Check sheet for the drawn part. Datum: minimum x, y, z corner. Units: mm. A direction names the side the tool comes from. Coordinates: 2 decimals unless noted, no trailing zeros. Loops run counter-clockwise (first coordinate to the right, second up) from the corner with the lowest first, then second, coordinate; pieces in that order, holes last.
Q1. Sectioned sample at C-C (x = 83). Enter the section's corners in (y, z).
Q2. Access from +Z, -Z, +X, -X, +Y, -Y to the whole of each face (thin tool, end or side, straight path). Record for the marked faces 5, 6 and 7.
Q3. Sectioned sample at D-D (x = 43.5). Enter the section's corners in (y, z).
Q4. Sectioned sample at A-A (z = 4). Enter the section's corners in (x, y), then the cut area to 3 significant figures.
Q5. Sectioned sample at B-B (y = 16.5). Enter the section's corners in (x, z), then the cut area to 3 significant figures.
Q6. Mould release check, pull along Z, two halves, no side actions. Record for the marked faces 1, 2, 3 and 4: +Z half, -Z half, draft (parallel to the pull), parting line (faces both ways), or undercut.
Q7. Material ranges on probe 1 along X at (y, z) = (1.3, 59); probe 2 along Z at (x, y) = (83, 1.75); probe 3 along Z at (x, y) = (73.5, 5.5), recorded low to high.
Q8. Go/stop test with flat-tipped pins: P1, Ø2.5, axis at x = 33.5, z = 4.5, coming from the +Y side; P2, Ø12, axis at y = 7.5, z = 49.5, coming from the -X side; P3, Ø1, axis at x = 68, y = 9, coming from the +Z side; P4, Ø8, axis at x = 38, z = 27, coming from the -Y side. Record where each tip stops, or that it passes through.
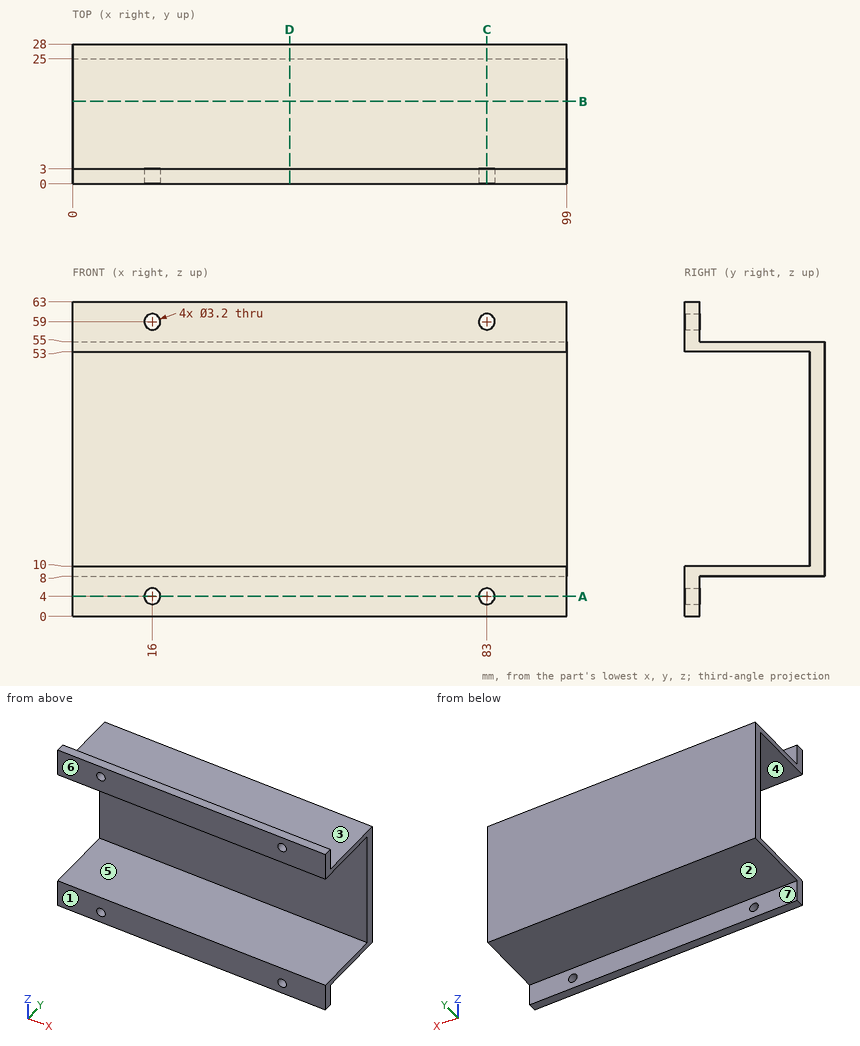
Geometry check:
1. outline: (0, 0) - (3, 0) - (3, 2.4) - (0, 2.4) - close; (0, 5.6) - (3, 5.6) - (3, 8) - (28, 8) - (28, 55) - (3, 55) - (3, 57.4) - (0, 57.4) - (0, 53) - (25, 53) - (25, 10) - (0, 10) - close; (0, 60.6) - (3, 60.6) - (3, 63) - (0, 63) - close
2. face 5: +X, -X, -Y
2. face 6: +Z, -Z, +X, -X, -Y
2. face 7: -Z, +X, -X, +Y
3. outline: (0, 0) - (3, 0) - (3, 8) - (28, 8) - (28, 55) - (3, 55) - (3, 63) - (0, 63) - (0, 53) - (25, 53) - (25, 10) - (0, 10) - close
4. outline: (0, 0) - (14.4, 0) - (14.4, 3) - (0, 3) - close; (17.6, 0) - (81.4, 0) - (81.4, 3) - (17.6, 3) - close; (84.6, 0) - (99, 0) - (99, 3) - (84.6, 3) - close
4. area: 278 mm2
5. outline: (0, 8) - (99, 8) - (99, 10) - (0, 10) - close; (0, 53) - (99, 53) - (99, 55) - (0, 55) - close
5. area: 396 mm2
6. face 1: draft
6. face 2: -Z half
6. face 3: +Z half
6. face 4: undercut
7. probe 1: x = 0 to 14.4, 17.6 to 81.4, 84.6 to 99
7. probe 2: z = 0 to 2.4, 5.6 to 10, 53 to 57.4, 60.6 to 63
7. probe 3: z = 8 to 10, 53 to 55
8. P1: stops at y = 3
8. P2: stops at x = 0
8. P3: stops at z = 55
8. P4: stops at y = 25
